```python
from build123d import *

# Parameters (mm, degrees)
F0_R     = 2.9
F1_DEPTH = 2
F2_R     = 1.9
F3_DEPTH = 12.55
F5_DEPTH = 2
F7_DEPTH = 25
F8_SIZE  = 0.5
F9_DEPTH = 25


# Not quite as in the source:
# - a feature names something its author has since deleted; it is built from what else it names


with BuildPart() as f1:
    # F0 (on Top) → F1 (new body)
    with BuildSketch(Plane.XY):
        with Locations((-52.0645752549, 27.8050955385)):
            Circle(F0_R)
    extrude(amount=F1_DEPTH)

    # F2 (on face) → F3 (join)
    with BuildSketch(Plane.XY.offset(2)):
        with Locations((-52.0645752549, 27.8050955385)):
            Circle(F2_R)
    extrude(amount=F3_DEPTH)

    # F4 (on face) → F5 (join)
    with BuildSketch(Plane.XY.offset(14.55)):
        with BuildLine():
            Line((-52.0645752549, 29.7050955385), (-54.2554654849, 29.7050955385))
            ThreePointArc((-54.2554654849, 29.7050955385), (-54.9645752549, 27.8050955385), (-54.2554654849, 25.9050955385))
            Line((-54.2554654849, 25.9050955385), (-52.0645752549, 25.9050955385))
            ThreePointArc((-52.0645752549, 25.9050955385), (-53.9645752549, 27.8050955385), (-52.0645752549, 29.7050955385))
        make_face()
        with BuildLine():
            ThreePointArc((-50.1645752549, 27.8050955385), (-50.7210723707, 29.1485984228), (-52.0645752549, 29.7050955385))
            ThreePointArc((-52.0645752549, 29.7050955385), (-53.9645752549, 27.8050955385), (-52.0645752549, 25.9050955385))
            ThreePointArc((-52.0645752549, 25.9050955385), (-50.7210723707, 26.4615926542), (-50.1645752549, 27.8050955385))
        make_face()
        with BuildLine():
            ThreePointArc((-49.8736850249, 25.9050955385), (-49.347630126, 26.7910890462), (-49.1645752549, 27.8050955385))
            ThreePointArc((-49.1645752549, 27.8050955385), (-49.347630126, 28.8191020308), (-49.8736850249, 29.7050955385))
            Line((-49.8736850249, 29.7050955385), (-52.0645752549, 29.7050955385))
            ThreePointArc((-52.0645752549, 29.7050955385), (-50.7210723707, 29.1485984228), (-50.1645752549, 27.8050955385))
            ThreePointArc((-50.1645752549, 27.8050955385), (-50.7210723707, 26.4615926542), (-52.0645752549, 25.9050955385))
            Line((-52.0645752549, 25.9050955385), (-49.8736850249, 25.9050955385))
        make_face()
    extrude(amount=F5_DEPTH)

    # F6 (on face) + F5_face1 (on face) → F7 (cut)
    with BuildSketch(Plane.XZ.offset(-25.9050955385)):
        with BuildLine():
            ThreePointArc((-53.0603808121, 16.3889640887), (-52.6208294658, 16.5013745209), (-52.1697451564, 16.55))
            Line((-52.1697451564, 16.55), (-53.0603808121, 16.55))
            Line((-53.0603808121, 16.55), (-53.0603808121, 16.3889640887))
        make_face()
        with BuildLine():
            Line((-51.0603808121, 16.55), (-51.9418670563, 16.55))
            ThreePointArc((-51.9418670563, 16.55), (-51.4955264095, 16.5022285059), (-51.0603808121, 16.3919996636))
            Line((-51.0603808121, 16.3919996636), (-51.0603808121, 16.55))
        make_face()
        with BuildLine():
            Line((-51.0603808121, 16.55), (-51.0603808121, 16.3919996636))
            ThreePointArc((-51.0603808121, 16.3919996636), (-50.428025883, 16.1031256959), (-49.8736850249, 15.6835698131))
            Line((-49.8736850249, 15.6835698131), (-49.8736850249, 16.55))
            Line((-49.8736850249, 16.55), (-51.0603808121, 16.55))
        make_face()
        with BuildLine():
            Line((-49.1058061063, 16.5520446822), (-52.0558061063, 16.5520446822))
            ThreePointArc((-52.0558061063, 16.5520446822), (-51.9988274089, 16.5515334705), (-51.9418670563, 16.55))
            Line((-51.9418670563, 16.55), (-51.0603808121, 16.55))
            Line((-51.0603808121, 16.55), (-49.8736850249, 16.55))
            Line((-49.8736850249, 16.55), (-49.8736850249, 15.6835698131))
            ThreePointArc((-49.8736850249, 15.6835698131), (-49.4281162504, 15.1596303152), (-49.1058061063, 14.5520446822))
            Line((-49.1058061063, 14.5520446822), (-49.1058061063, 16.5520446822))
        make_face()
        with BuildLine():
            Line((-54.2554654849, 16.55), (-54.2554654849, 15.666854741))
            ThreePointArc((-54.2554654849, 15.666854741), (-53.6981031241, 16.0944069239), (-53.0603808121, 16.3889640887))
            Line((-53.0603808121, 16.3889640887), (-53.0603808121, 16.55))
            Line((-53.0603808121, 16.55), (-54.2554654849, 16.55))
        make_face()
        with BuildLine():
            Line((-52.0558061063, 16.5520446822), (-55.0058061063, 16.5520446822))
            Line((-55.0058061063, 16.5520446822), (-55.0058061063, 14.5520446822))
            ThreePointArc((-55.0058061063, 14.5520446822), (-54.6902791648, 15.1495936288), (-54.2554654849, 15.666854741))
            Line((-54.2554654849, 15.666854741), (-54.2554654849, 16.55))
            Line((-54.2554654849, 16.55), (-53.0603808121, 16.55))
            Line((-53.0603808121, 16.55), (-52.1697451564, 16.55))
            ThreePointArc((-52.1697451564, 16.55), (-52.1127848038, 16.5515334705), (-52.0558061063, 16.5520446822))
        make_face()
        Polygon((-52.0645752549, 14.55), (-53.0603808121, 14.55), (-53.0603808121, 7.8), (-51.0603808121, 7.8), (-51.0603808121, 13.8), (-51.0603808121, 14.55), align=None)
    with BuildSketch(Plane(origin=(-52.0645752549, 29.7050955385, 15.55), x_dir=(-1, 0, 0), z_dir=(0, 1, 0))):
        Polygon((-2.19089023, 1), (-2.19089023, -1), (0, -1), (2.19089023, -1), (2.19089023, 1), align=None)
    extrude(amount=-F7_DEPTH, dir=(0, -1, 0), mode=Mode.SUBTRACT)

    # F8
    f8_edges = [f1.edges().sort_by_distance(p)[0] for p in [
        (-54.964575, 27.805096, 2),
    ]]
    chamfer(f8_edges, length=F8_SIZE)

    # F6 (on face) → F9 (cut)
    with BuildSketch(Plane.XZ.offset(-25.9050955385)):
        with BuildLine():
            ThreePointArc((-51.0603808121, 16.3919996636), (-51.4955264095, 16.5022285059), (-51.9418670563, 16.55))
            Line((-51.9418670563, 16.55), (-52.1697451564, 16.55))
            ThreePointArc((-52.1697451564, 16.55), (-52.6208294658, 16.5013745209), (-53.0603808121, 16.3889640887))
            Line((-53.0603808121, 16.3889640887), (-53.0603808121, 14.5520446822))
            Line((-53.0603808121, 14.5520446822), (-53.0603808121, 14.55))
            Line((-53.0603808121, 14.55), (-52.0645752549, 14.55))
            Line((-52.0645752549, 14.55), (-51.0603808121, 14.55))
            Line((-51.0603808121, 14.55), (-51.0603808121, 14.5520446822))
            Line((-51.0603808121, 14.5520446822), (-51.0603808121, 16.3919996636))
        make_face()
        Polygon((-52.0645752549, 14.55), (-53.0603808121, 14.55), (-53.0603808121, 7.8), (-51.0603808121, 7.8), (-51.0603808121, 13.8), (-51.0603808121, 14.55), align=None)
    extrude(amount=-F9_DEPTH, mode=Mode.SUBTRACT)


solid = f1.part
```
Work out the finished part from the listing and answer in its coordinate system (mm). A direction names the side the tool comes from. Round coordinates to 2 decimals unless told otherwise and drop trailing zeros. Loops run counter-clockwise (first coordinate to the right, second up) from the corner with the lowest first, then second, coordinate; pieces in that order, holes last. Notation, with made-up numbers: (55, 73) -> (60, 73) arc R34 cw to (60, 104) -> close; hole circle Ø7 at (66.5, 5.5). An arc over 180 degrees is marked (long way). Write each question's results on one line, items separated by ' | '. Start each with the question number.
1. Given pin 1 Ø0.9 at (x, z) = (-50.5, 15) entering from +Y; pin 2 Ø0.6 at (x, z) = (-50.5, 15) entering from -Y; pin 3 Ø0.6 at (x, y) = (-52, 27) entering from +Z, each flat-ended and moving along its own axis, determine where each tip first touches the part or whether it passes through.
2. For a pull along Z with two mould halves and no side action, classify faces 6 (the face through (-50.5, 25.905, 15.3)), 7 (the face through (-52, 28, 0)), 8 (the face through (-50, 28, 14.55)) as +Z half, -Z half, draft (parallel to the pull), parting line (faces both ways), or undercut.
3. A tool of negligible diameter and unlimited length cuts with its end or side. For faces 1 (the face through (-50.5, 29.705, 15.3)), 2 (the face through (-54, 25.905, 15)), 3 (the face through (-51.06, 28, 12)), 4 (the face through (-54.2, 27.8, 14.55)), 5 (the face through (-53.465, 29.089, 8.187)), from which of +Z, -Z, +X, -X, +Y, -Y can it reach the whole face along a straight path? Write none if from no direction.
4. Find the intervals of material crossed by probe 1 along X at (y, z) = (27.9, 5.5); probe 2 along X at (y, z) = (28.9, 10.5); probe 3 along X at (y, z) = (26.8, 14), in increasing order. Write a range as from..to.
5. Section A-A (z = 10.5) is taken. Determine the outline of the cut face in (x, y), plus the area to 3 significant figures.
Evaluation:
1) pin 1: stops at y = 29.71 | pin 2: stops at y = 25.91 | pin 3: stops at z = 7.8
2) face 6: draft | face 7: -Z half | face 8: undercut
3) face 1: +Z, +X, -X, +Y | face 2: +Z, +X, -X, -Y | face 3: +Z, +Y, -Y | face 4: -X | face 5: none
4) probe 1: x = -53.96..-50.17 | probe 2: x = -53.62..-53.06, -51.06..-50.51 | probe 3: x = -53.68..-53.06, -51.06..-50.45
5) outline: (-53.06, 26.19) -> (-53.06, 29.42) arc R1.9 ccw to start; (-51.06, 26.19) arc R1.9 ccw to (-51.06, 29.42) -> close | area: 4.11 mm2
